The listing builds one solid part. Answer for the finished solid, in the listing's coordinates (mm). Face numbers are marked on the shaded views. Round coordinates to 2 decimals unless told otherwise and drop trailing zeros. Write each loop counter-clockwise with the first axis right and the second up, starting at its lowest first coordinate (ties: lowest second). Pieces come first, ordered by that corner, then holes. Notation, with made-up numbers: (5, 35) - (50, 35) arc R13 ccw to (50, 54) - close; hole circle Ø5 at (6.5, 14). An arc over 180 degrees is marked (long way). Use a Markdown table: item, result. Add a question column.
1) Determine the mould class of the marked faces 1, 2 and 3 for opening direction X: +X half, -X half, draft (parallel to the pull), parting line (faces both ways), or undercut.
2) A cutting plane is placed at D-D (z = 38.25). Give the vertices of the cut face in (x, y).
3) A cutting plane is placed at B-B (z = 28.75). Give the vertices of the cut face in (x, y).
4) This flat-tipped pin is pushed along its axis until it touches: P1, Ø5, axis at y = -11.5, z = 35, coming from the +X side. Where does it stop, or does it pass through?
5) Find the intervals of material crossed by probe 1 along Z at (x, y) = (-7, -2); probe 2 along Z at (x, y) = (29, -41.5); probe 3 along Z at (x, y) = (-4, -40), in increasing order. Write a range as from..to.
6) A cutting plane is placed at A-A (x = -2.5). Give the vertices of the cut face in (y, z).
7) A cutting plane is placed at C-C (y = -23). Give the vertices of the cut face in (x, z).
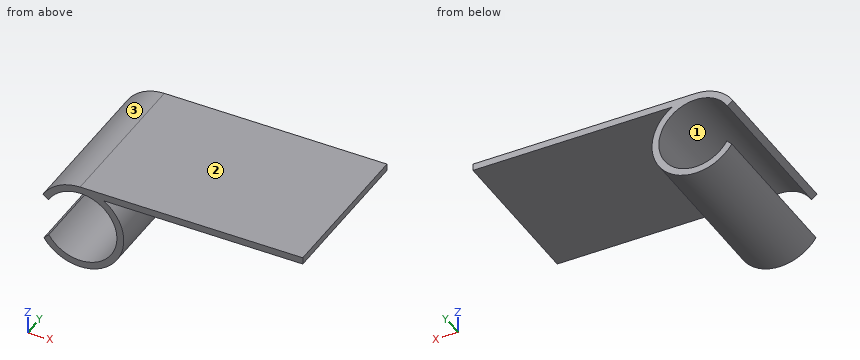
```python
from build123d import *

# Parameters (mm, degrees)
F1_DEPTH = 46


with BuildPart() as f1:
    # F0 (on Front) → F1 (new body)
    with BuildSketch(Plane.XZ):
        with BuildLine():
            ThreePointArc((-15.733881, 43.227494), (4.28348, 37.915884), (-15.594438, 32.104143))
            Line((-15.594438, 32.104143), (-17.024878, 30.635102))
            ThreePointArc((-17.024878, 30.635102), (2.671941, 28.889199), (0.389979, 48.531132))
            Line((0.389979, 48.531132), (58.534325, 48.531132))
            Line((58.534325, 48.531132), (58.534325, 50.531132))
            Line((58.534325, 50.531132), (-6.465675, 50.531132))
            ThreePointArc((-6.465675, 50.531132), (-12.661991, 48.924209), (-17.296424, 44.508492))
            Line((-17.296424, 44.508492), (-15.733881, 43.227494))
        make_face()
    extrude(amount=F1_DEPTH)


solid = f1.part
```
Entries:
| question | item | result |
|---|---|---|
| 1 | face 1 | undercut |
| 1 | face 2 | draft |
| 1 | face 3 | -X half |
| 2 | outline | (4.27, -46) - (6.28, -46) - (6.28, 0) - (4.27, 0) - close |
| 3 | outline | (-15.47, -46) - (-12.3, -46) - (-12.3, 0) - (-15.47, 0) - close; (-0.63, -46) - (2.53, -46) - (2.53, 0) - (-0.63, 0) - close |
| 4 | P1 | stops at x = 6.28 |
| 5 | probe 1 | z = 25.04..27.04, 48.52..50.52 |
| 5 | probe 2 | z = 48.53..50.53 |
| 5 | probe 3 | z = 25.27..27.32, 48.24..50.53 |
| 6 | outline | (-46, 25.66) - (0, 25.66) - (0, 27.79) - (-46, 27.79) - close; (-46, 47.77) - (0, 47.77) - (0, 50.53) - (-46, 50.53) - close |
| 7 | outline | (-17.3, 44.51) - (-15.73, 43.23) arc R10.75 cw (long way) to (-15.59, 32.1) - (-17.02, 30.64) arc R12.75 ccw (long way) to (0.39, 48.53) - (58.53, 48.53) - (58.53, 50.53) - (-6.47, 50.53) arc R12.75 ccw to start |
